The model under review builds one solid part; all positions refer to its coordinate system, in mm. Face numbers are marked on the shaded views. Give positions to 0.01 mm unless a question says otherwise; leave off trailing zeros. Order: outer loops, then holes, each group sorted by start corner. A loop starts at its lowest first (then second) coordinate and runs counter-clockwise, first axis right, second up. Notation, with made-up numbers: (81.5, -3.75) - (115.5, -3.75) arc R10 ccw to (115.5, 15.25) - close; hole circle Ø2 at (25.5, -18). An arc over 180 degrees is marked (long way). Use CSV: the item, a comma, the result in double quotes.
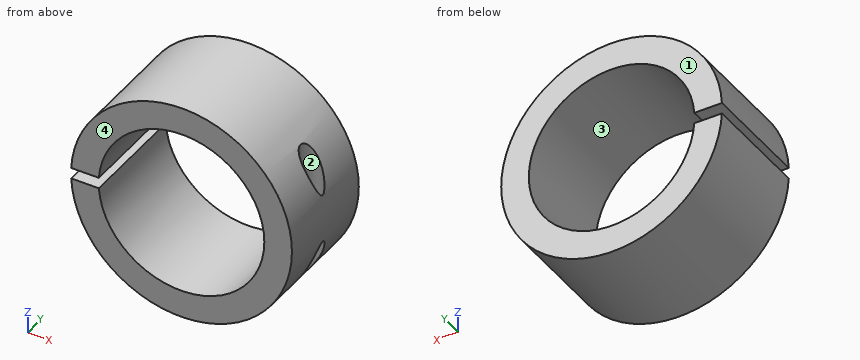
Autodesk Inventor part; units mm, degrees
ref_plane "工作平面1" through (0, 0, 3) normal (0, 0, 1) x (1, 0, 0)
ref_plane "YZ Plane" through (0, 0, 0) normal (1, 0, 0) x (0, 1, 0)
ref_plane "XZ Plane" through (0, 0, 0) normal (0, 1, 0) x (-1, 0, 0)
sketch "草圖1" plane through (0, 0, 0) normal (0, 1, 0) x (-1, 0, 0)
  circle A0 centre (0, 0) radius 15
  circle A1 centre (0, 0) radius 20
  dimension "d0" = 30
  dimension "d1" = 5
extrude "擠出1" add sketch "草圖1" along normal mid plane 20
sketch "草圖2" plane through (0, 0, 0) normal (0, 0, 1) x (1, 0, 0)
  circle A0 centre (0, 0) radius 3
  dimension "d4" = 6
sketch "草圖3" plane through (0, 0, 0) normal (0, 0, 1) x (1, 0, 0)
  line L0 (-20, -10) -> (20, -10)
  line L1 (20, 10) -> (-20, 10)
  circle A0 centre (17.5034, 0) radius 1
  line L2 (20, 10) -> (20, -10)
  line L3 (20, -10) -> (20, 10)
  line L4 (20, 10) -> (-20, 10)
  line L5 (15.0068, 10) -> (20, 10)
  point P0 (0, 0)
  point P1 (20, 0)
  point P2 (17.5034, 10)
  dimension "d5" = 2
extrude "擠出2" cut sketch "草圖3" along normal through all both and the other way through all
sketch "草圖4" plane through (0, 0, 0) normal (0, 1, 0) x (-1, 0, 0)
  circle A0 centre (0, 0) radius 20
  circle A1 centre (0, 0) radius 15
  circle A2 centre (0, 0) radius 20
  line L0 (19.975, -1) -> (14.9666, -1)
  circle A3 centre (0, 0) radius 15
  line L1 (28, 0) -> (-28, 0)
  line L2 (19.975, 1) -> (14.9666, 1)
  dimension "d8" = 1
extrude "擠出3" cut sketch "草圖4" along normal through all both and the other way through all contours L1 A1 L2 A0 | A0 L0 A1 L1 picked at (16.6568, 0.5558) picked at (16.6568, -0.5558)
ref_plane "工作平面1" through (0, 0, 3) normal (0, 0, 1) x (1, 0, 0)
sketch "草圖5" plane through (0, 0, 3) normal (0, 0, 1) x (1, 0, 0)
  line L0 (-19.975, 10) -> (-19.975, -10)
  line L1 (-19.975, -10) -> (-19.975, -10)
  line L2 (-19.975, -10) -> (-19.975, 10)
  line L3 (-19.975, 10) -> (-19.975, 10)
  spline S0 degree 5 poles (16.5034, 0) (16.5037, -0.3304) (16.6391, -0.6617) (16.9151, -0.9151) (17.5618, -1.1213) (18.1683, -0.8385) (18.3912, -0.5976) (18.6137, -0.0031) (18.395, 0.593) (18.1721, 0.8363) (17.5647, 1.1217) (16.9159, 0.9158) (16.6393, 0.6625) (16.5037, 0.3307) (16.5034, 0) knots 0 0 0 0 0 0 0.26304 0.26304 0.26304 0.499355 0.499355 0.499355 0.736707 0.736707 0.736707 1 1 1 1 1 1
  line L4 (19.7737, 10) -> (19.7737, -10)
  line L5 (19.7737, -10) -> (14.6969, -10)
  line L6 (14.6969, -10) -> (14.6969, 10)
  line L7 (14.6969, 10) -> (19.7737, 10)
  circle A0 centre (17.5034, 0) radius 1
  line L8 (-19.7737, -10) -> (-19.7737, 10)
  line L9 (-19.7737, 10) -> (-14.6969, 10)
  line L10 (-14.6969, 10) -> (-14.6969, -10)
  line L11 (-14.6969, -10) -> (-19.7737, -10)
  line L12 (14.6969, 10) -> (19.7737, 10)
  line L13 (19.7737, 10) -> (19.7737, -10)
  line L14 (19.7737, -10) -> (14.6969, -10)
  line L15 (14.6969, -10) -> (14.6969, 10)
  circle A1 centre (17.5034, 0) radius 2
  point P0 (0, 0)
  point P1 (18.3303, -0.5624)
  point P2 (19.7737, 0)
  point P3 (17.2353, 10)
  dimension "d15" = 4
extrude "擠出5" cut sketch "草圖5" along normal through all both and the other way through all contours A1
properties part number "0311_練習2"
Item 1: Clearance check with flat-ended pins moving along their axes: pin 1 (2.5 mm diameter, centred on x = -17, y = -4.5, fed in from +Z); pin 2 (4 mm diameter, centred on x = -18, y = 4, fed in from -Z); pin 3 (1.5 mm diameter, centred on x = 4.5, y = 3, fed in from -Z); pin 4 (8 mm diameter, centred on y = 2.5, z = 0.5, fed in from -X) (3 decimals). State where each tip first meets the part, or that it passes through.
Results list:
pin 1,"stops at z = 12.33"
pin 2,"stops at z = -12"
pin 3,"stops at z = -19.65"
pin 4,"stops at x = -19.975"
Item 2: Take a section at C-C, the plane y = 0. Give the boundary of the cut face in (x, z) (3 decimals).
Results list:
outline,"(-19.975, -1) arc R20 ccw to (15.503, -12.635) - (15.503, 12.635) arc R20 ccw to (-19.975, 1) - (-14.967, 1) arc R15 cw (long way) to (-14.967, -1) - close; (19.503, -4.429) arc R20 ccw to (19.503, 4.429) - close"
Item 3: Take a section at D-D, the plane z = 0. Give the boundary of the cut face in (x, y), and give its area (3 significant figures).
Results list:
outline,"(15, -10) - (20, -10) - (20, 10) - (15, 10) - close; hole circle Ø4 at (17.5, 0)"
area,"87.4 mm2"
Item 4: Wall thickness on L1, parallel to Z at x = 0, y = -6; L2, parallel to X at y = 0, z = 1.5; L3, parallel to X at y = -2.25, z = 6: over which ranges is each line inside the solid? List them lowest first.
Results list:
L1,"z = -20 to -15, 15 to 20"
L2,"x = -19.94 to -14.92, 14.92 to 15.5, 19.5 to 19.94"
L3,"x = -19.08 to -13.75, 13.75 to 19.08"
Item 5: Mouldability with a two-part tool opening along Y and no side actions: class the marked faces 1, 2, 3 and 4 as pulls with the +Y half, pulls with the -Y half, needs draft (parallel to the pull), parting line crosses it, or undercut.
Results list:
face 1,"pulls with the +Y half"
face 2,"undercut"
face 3,"needs draft"
face 4,"pulls with the -Y half"
Item 6: Take a section at A-A, the plane x = 0. Give the boundary of the cut face in (y, z), and give its area (3 significant figures).
Results list:
outline,"(-10, -20) - (10, -20) - (10, -15) - (-10, -15) - close; (-10, 15) - (10, 15) - (10, 20) - (-10, 20) - close"
area,"200 mm2"
Item 7: Take a section at B-B, the plane z = 11.5. Give the boundary of the cut face in (x, y).
Results list:
outline,"(-16.36, -10) - (-9.63, -10) - (-9.63, 10) - (-16.36, 10) - close; (9.63, -10) - (16.36, -10) - (16.36, -1.64) arc R2 cw to (16.36, 1.64) - (16.36, 10) - (9.63, 10) - close"
